For this review, take the finished solid that the model builds, in its own axes (mm). Coordinates: 2 decimals unless noted, no trailing zeros. Loops run counter-clockwise (first coordinate to the right, second up) from the corner with the lowest first, then second, coordinate; pieces in that order, holes last. Notation, with made-up numbers: M 51,56 L 95,56 A9 ccw 95,68 Z; hole C -14.5,28 d5. An arc over 180 degrees is marked long. Use one line per item in the form item = value.
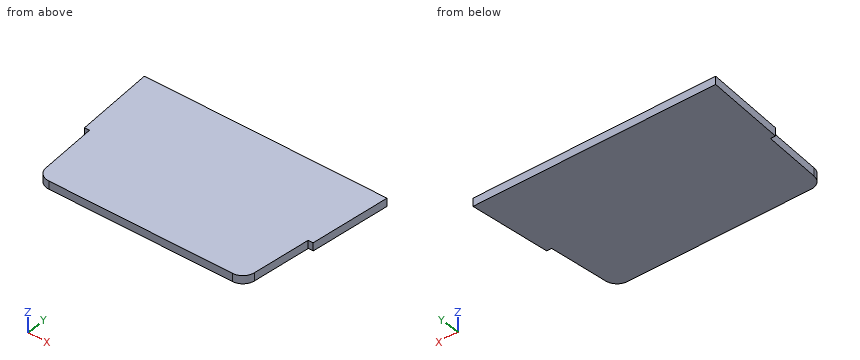
```python
from build123d import *

# Parameters (mm, degrees)
F1_DEPTH = 3.175
F2_R     = 5


with BuildPart() as f1:
    # F0 (on Top) → F1 (new body)
    with BuildSketch(Plane.XY):
        Polygon((48.75, 14.636084), (-48.75, 14.636084), (-45.944906, -17.488916), (-43.944906, -17.488916), (-41.5, -45.488916), (0, -45.488916), (41.5, -45.488916), (43.944906, -17.488916), (45.944906, -17.488916), align=None)
    extrude(amount=F1_DEPTH)

    # F2
    f2_edges = [f1.edges().sort_by_distance(p)[0] for p in [
        (-41.5, -45.488916, 1.5875),
        (41.5, -45.488916, 1.5875),
    ]]
    fillet(f2_edges, radius=F2_R)


solid = f1.part
```
1. Consider section B-B on y = 0. Write out the cut boundary in (x, z) (3 decimals), plus the area to 3 significant figures.
Computed values:
outline = M -47.472,0 L 47.472,0 L 47.472,3.175 L -47.472,3.175 Z
area = 301 mm2
2. Consider section A-A on z = 0.55. Write out the cut boundary in (x, y).
Computed values:
outline = M -48.75,14.64 L -45.94,-17.49 L -43.94,-17.49 L -41.9,-40.92 A5 ccw -36.92,-45.49 L 36.92,-45.49 A5 ccw 41.9,-40.92 L 43.94,-17.49 L 45.94,-17.49 L 48.75,14.64 Z
3. Consider section C-C on x = -40.5. Write out the cut boundary in (y, z) (3 decimals).
Computed values:
outline = M -43.977,0 L 14.636,0 L 14.636,3.175 L -43.977,3.175 Z
4. Wall thickness on line 1 along X through (y, z) = (1.5, 1); line 2 along X through (y, z) = (-32.5, 1.05); line 3 along Y through (x, z) = (-39.5, 1.65): over which ranges is each line inside the solid? List them lowest first. Write a range as from..to.
Computed values:
line_1 = -47.6..47.6
line_2 = -42.63..42.63
line_3 = -44.77..14.64
